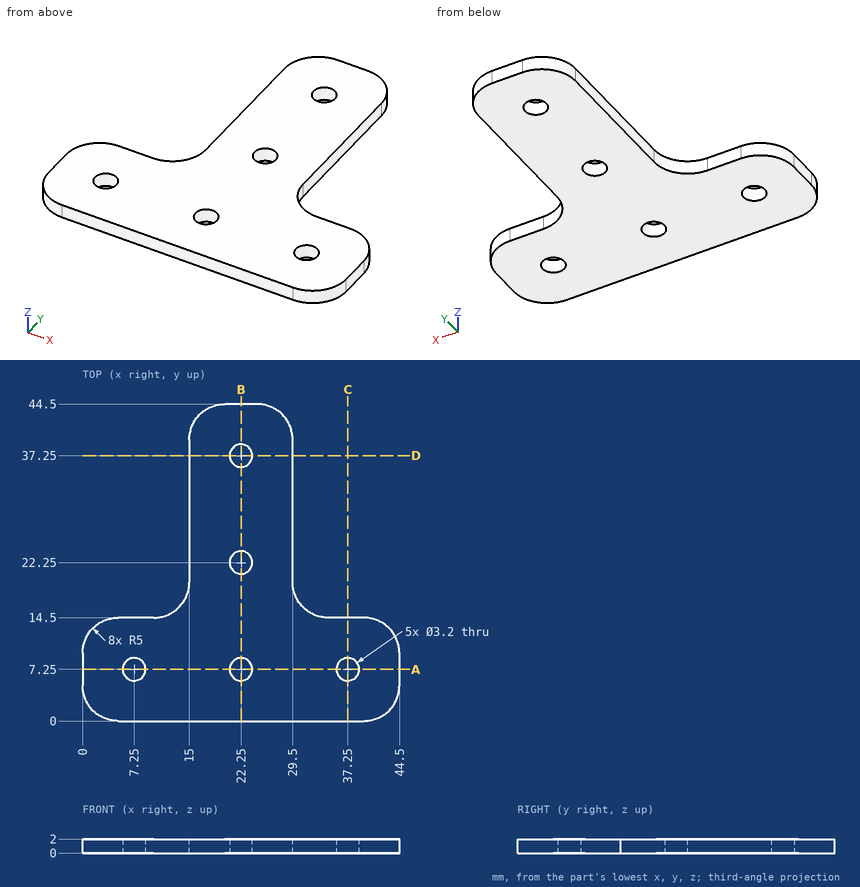
Job drawing, mm, ordinate dimensions from the low corner. One solid piece. Round coordinates to 2 decimals unless told otherwise and drop trailing zeros. Write each loop counter-clockwise with the first axis right and the second up, starting at its lowest first coordinate (ties: lowest second). Pieces come first, ordered by that corner, then holes.
1) Band-saw the part on D-D, the plane y = 37.25. List the corners of the cut face in (x, z).
2) Band-saw the part on A-A, the plane y = 7.25. List the corners of the cut face in (x, z), and give its area (3 significant figures).
3) Band-saw the part on C-C, the plane x = 37.25. List the corners of the cut face in (y, z), and give its area (3 significant figures).
4) Drill centre lines: probe 1 along Y at (x, z) = (22.25, 1); probe 2 along Y at (x, z) = (7.25, 0.95); probe 3 along X at (y, z) = (8.5, 1.1). Where is each one in solid material? Low to high.
5) Pin check, flat tips, straight feed: pin 1 (1.9 mm diameter, centred on x = 37.25, y = 7.25, fed in from +Z); pin 2 (0.6 mm diameter, centred on x = 37, z = 1, fed in from +Y). Stop position of each tip, or through.
Ans:
1. outline: (15, 0) - (20.65, 0) - (20.65, 2) - (15, 2) - close; (23.85, 0) - (29.5, 0) - (29.5, 2) - (23.85, 2) - close
2. outline: (0, 0) - (5.65, 0) - (5.65, 2) - (0, 2) - close; (8.85, 0) - (20.65, 0) - (20.65, 2) - (8.85, 2) - close; (23.85, 0) - (35.65, 0) - (35.65, 2) - (23.85, 2) - close; (38.85, 0) - (44.5, 0) - (44.5, 2) - (38.85, 2) - close
2. area: 69.8 mm2
3. outline: (0, 0) - (5.65, 0) - (5.65, 2) - (0, 2) - close; (8.85, 0) - (14.5, 0) - (14.5, 2) - (8.85, 2) - close
3. area: 22.6 mm2
4. probe 1: y = 0 to 5.65, 8.85 to 20.65, 23.85 to 35.65, 38.85 to 44.5
4. probe 2: y = 0 to 5.65, 8.85 to 14.5
4. probe 3: x = 0 to 6.25, 8.25 to 21.25, 23.25 to 36.25, 38.25 to 44.5
5. pin 1: passes through
5. pin 2: stops at y = 14.5
